```python
from build123d import *

# Parameters (mm, degrees)
F0_W     = 76.2
F0_H     = 508
F1_DEPTH = 76.2
F3_DEPTH = 50.8


with BuildPart() as f1:
    # F0 (on Front) → F1 (new body)
    with BuildSketch(Plane.XZ):
        Rectangle(F0_W, F0_H)
    extrude(amount=F1_DEPTH)

    # F2 (on face) → F3 (cut)
    with BuildSketch(Plane.XY.offset(254)):
        Polygon((12.7, 0), (-12.7, 0), (-12.7, -25.4), (-38.1, -25.4), (-38.1, -50.8), (-12.7, -50.8), (-12.7, -76.2), (12.7, -76.2), (12.7, -50.8), (38.1, -50.8), (38.1, -25.4), (12.7, -25.4), align=None)
    extrude(amount=-F3_DEPTH, mode=Mode.SUBTRACT)


solid = f1.part
```
Geometry: final body of the model. Coordinates: model frame, mm. A direction names the side the tool comes from. Give positions to 0.01 mm unless a question says otherwise; leave off trailing zeros. Loops run counter-clockwise (first coordinate to the right, second up) from the corner with the lowest first, then second, coordinate; pieces in that order, holes last. Notation, with made-up numbers: (-34, -30) - (-26, -30) arc R28 ccw to (-26, 3) - close; hole circle Ø11 at (-13.75, 73.5). An arc over 180 degrees is marked (long way). Answer as CSV lines item,"result". Start each with the question number.
(1) Section query C-C (y = -6). Output: boundary loops of the cut face in (x, z), and give its area (3 significant figures).
(2) Ray query, line 1 along Z through (x, y) = (27, -32.5); line 2 along Y through (x, z) = (-33.5, 212). Return the intervals inside material, ascending. Write a range as [from, to].
(3) Section query D-D (y = -45.5). Output: boundary loops of the cut face in (x, z).
(4) Mould query, pull axis Y, two halves, no side actions, for faces 1 (the face through (-1, -38, 203.2)), 2 (the face through (12.7, -64, 229)), 3 (the face through (-1, -76.2, 4)), 4 (the face through (-26, -50.8, 229)). Classes: +Y half, -Y half, draft (parallel to the pull), parting line (faces both ways), or undercut.
(5) Section query A-A (z = 217). Output: boundary loops of the cut face in (x, y), and give its area (3 significant figures).
(6) Pin query (flat end, axial travel): P1, Ø2, axis at x = -16.5, z = -136.5, coming from the +Y side. Return the tip coordinate at first contact, or that it passes through.
(7) Reachability of faces 5 (the face through (25, -13, 254)), 6 (the face through (12.7, -13, 229)), 7 (the face through (26, -25.4, 229)) from +Z, -Z, +X, -X, +Y, -Y: full face, straight path, thin tool, end or side. Return the list, or none.
(8) Section query B-B (x = -33). Output: boundary loops of the cut face in (y, z).
Worked answers:
1,outline,"(-38.1, -254) - (38.1, -254) - (38.1, 254) - (12.7, 254) - (12.7, 203.2) - (-12.7, 203.2) - (-12.7, 254) - (-38.1, 254) - close"
1,area,"37,400 mm^2"
2,line 1,"z = [-254, 203.2]"
2,line 2,"y = [-76.2, -50.8], [-25.4, 0]"
3,outline,"(-38.1, -254) - (38.1, -254) - (38.1, 203.2) - (-38.1, 203.2) - close"
4,face 1,"undercut"
4,face 2,"draft"
4,face 3,"-Y half"
4,face 4,"undercut"
5,outline,"(-38.1, -76.2) - (-12.7, -76.2) - (-12.7, -50.8) - (-38.1, -50.8) - close; (-38.1, -25.4) - (-12.7, -25.4) - (-12.7, 0) - (-38.1, 0) - close; (12.7, -76.2) - (38.1, -76.2) - (38.1, -50.8) - (12.7, -50.8) - close; (12.7, -25.4) - (38.1, -25.4) - (38.1, 0) - (12.7, 0) - close"
5,area,"2,580 mm^2"
6,P1,"stops at y = 0"
7,face 5,"+Z, +X, -X, +Y, -Y"
7,face 6,"+Z, +Y, -Y"
7,face 7,"+Z, +X, -X"
8,outline,"(-76.2, -254) - (0, -254) - (0, 254) - (-25.4, 254) - (-25.4, 203.2) - (-50.8, 203.2) - (-50.8, 254) - (-76.2, 254) - close"
